from build123d import *

# Parameters (mm, degrees)
F1_DEPTH = 1
F2_W     = 18.6
F2_H     = 1
F3_DEPTH = 13
F4_R     = 2
F5_R     = 1


with BuildPart() as f1:
    # F0 (on Top) → F1 (new body)
    with BuildSketch(Plane.XY):
        Polygon((0, 67), (0, 0), (18.6, 0), (18.6, 67), (14.4, 70.8), (14.4, 79), (4.2, 79), (4.2, 70.8), align=None)
    extrude(amount=F1_DEPTH)

    # F2 (on Top) → F3 (join)
    with BuildSketch(Plane.XY):
        with Locations((5.9, -0.5)):
            Rectangle(F2_W, F2_H)
    extrude(amount=F3_DEPTH)

    # F4
    f4_edges = [f1.edges().sort_by_distance(p)[0] for p in [
        (18.6, 0, 0.5),
        (15.2, -0.5, 13),
        (-3.4, -0.5, 13),
        (14.4, 79, 0.5),
        (4.2, 79, 0.5),
    ]]
    fillet(f4_edges, radius=F4_R)

    # F5
    f5_edges = [f1.edges().sort_by_distance(p)[0] for p in [
        (7.6, 0, 1),
    ]]
    fillet(f5_edges, radius=F5_R)


solid = f1.part
Part model, mm, in its own coordinate system. A direction names the side the tool comes from. Coordinates: 2 decimals unless noted, no trailing zeros. Order: outer loops, then holes, each group sorted by start corner. A loop starts at its lowest first (then second) coordinate and runs counter-clockwise, first axis right, second up. Notation, with made-up numbers: M -4.75,68 L 3.25,68 A21 cw 3.25,79 Z; hole C 71,58.25 d2. An arc over 180 degrees is marked long. Use a Markdown table: item, result.
(1) Flat gauge pins, fed straight in: pin 1 (10 mm diameter, centred on x = 9, y = 31, fed in from +Z); pin 2 (1.1 mm diameter, centred on x = 16, z = 0.5, fed in from -Y); pin 3 (2 mm diameter, centred on y = 38, z = 1, fed in from -X); pin 4 (5 mm diameter, centred on y = 64, z = 5.5, fed in from -X). Where does each tip first touch, or does it go through?
A:
| item | result |
|---|---|
| pin 1 | stops at z = 1 |
| pin 2 | stops at y = 0 |
| pin 3 | stops at x = 0 |
| pin 4 | passes through |
(2) Probe L1, parallel to Z at x = 1.25, y = 23.5; L2, parallel to Y at x = 1, z = 2.5. List the from-to ranges inside material, lowest first.
A:
| item | result |
|---|---|
| L1 | z = 0 to 1 |
| L2 | y = -1 to 0 |
(3) Cut at A-A on x = 7.5. Write the cut outline in (y, z), then the cut area to 3 significant figures.
A:
| item | result |
|---|---|
| outline | M -1,0 L 79,0 L 79,1 L 1,1 A1 cw 0,2 L 0,13 L -1,13 Z |
| area | 92.2 mm^2 |
(4) Cut at D-D on x = 3.25. Write the cut outline in (y, z).
A:
| item | result |
|---|---|
| outline | M -1,0 L 69.94,0 L 69.94,1 L 1,1 A1 cw 0,2 L 0,13 L -1,13 Z |
(5) Cut at B-B on z = 3.75. Write the cut outline in (x, y), then the cut area to 3 significant figures.
A:
| item | result |
|---|---|
| outline | M -3.4,-1 L 15.2,-1 L 15.2,0 L -3.4,0 Z |
| area | 18.6 mm^2 |
(6) Cut at C-C on y = 50.5. Write the cut outline in (x, z).
A:
| item | result |
|---|---|
| outline | M 0,0 L 18.6,0 L 18.6,1 L 0,1 Z |
(7) Tool access for faces 1 (the flat face through (0, 34, 0.5)), 2 (the cylindrical face through (18, 0.57, 0.51)): list every direction of +Z, -Z, +X, -X, +Y, -Y with a clear straight run to the whole face (end or side of a thin tool).
A:
| item | result |
|---|---|
| face 1 | +Z, -Z, -X, +Y |
| face 2 | +Z, -Z, +X, -Y |
